from build123d import *


with BuildPart() as f1:
    # F0 (on Front) → F1 (revolve)
    with BuildSketch(Plane.XZ):
        Polygon((2.2225, 3.048), (2.2225, 0), (4.678082, 0), (4.826, 0.4064), (4.826, 1.143), (3.81, 1.143), (3.81, 1.778), (4.826, 4.569437), (4.826, 15.1384), (3.937, 16.3068), (3.937, 19.7104), (3.6068, 19.7104), (3.6068, 16.3068), (4.4958, 15.1384), (4.064, 4.064), (0.9398, 4.064), (0.9398, 3.048), align=None)
    revolve(axis=Axis((0, 0, 11.499301), (0, 0, 1)))


with BuildPart() as f2_1:
    # F2: copy of F1
    add(f1.part)


solid = f1.part
The model under review builds one solid part; all positions refer to its coordinate system, in mm. A direction names the side the tool comes from. Round coordinates to 2 decimals unless told otherwise and drop trailing zeros. Write each loop counter-clockwise with the first axis right and the second up, starting at its lowest first coordinate (ties: lowest second). Pieces come first, ordered by that corner, then holes. Notation, with made-up numbers: (69, 40.25) -> (97, 40.25) arc R17 ccw to (97, 62.25) -> close; hole circle Ø3 at (-4, 27). An arc over 180 degrees is marked (long way). Answer as a JSON object with one key per item and string values.
1. Clearance check with flat-ended pins moving along their axes: pin 1 (5 mm diameter, centred on y = -3.5, z = 5.5, fed in from +X); pin 2 (3 mm diameter, centred on x = 0, y = 0, fed in from +Z); pin 3 (1.5 mm diameter, centred on x = -3, z = 8, fed in from +Y); pin 4 (5 mm diameter, centred on x = 2.5, z = 4.5, fed in from -Y). State where each tip first meets the part, or that it passes through.
Results found:
{"pin 1": "stops at x = 4.72", "pin 2": "stops at z = 4.06", "pin 3": "stops at y = 4.27", "pin 4": "stops at y = -4.83"}
2. We need section C-C on z = 18. State the section outline as (x, y) points.
Results found:
{"outline": "circle Ø7.87 at (0, 0); hole circle Ø7.21 at (0, 0)"}
3. Machinability: for faces 5 (the face through (-0.48, -2.17, 1.5)), 6 (the face through (-0.83, -3.72, 1.46)), 7 (the face through (-3.83, -2.937, 9.928)), 8 (the face through (-0.853, -3.843, 18.032)), which of the approach directions +Z, -Z, +X, -X, +Y, -Y give a long, thin tool a straight path to every point of the face, cutting with its end or side? Answer none if there is none.
Results found:
{"face 5": "-Z", "face 6": "none", "face 7": "+Z, -Z", "face 8": "+Z"}
4. To check wall thickness, follow line 1 along Y through (x, z) = (0, 17.4); line 2 along Y through (x, z) = (1.5, 7.75); line 3 along Z through (x, y) = (0.75, 1.5). State the ranges of each line that lie inside material, in increasing order.
Results found:
{"line 1": "y = -3.94 to -3.61, 3.61 to 3.94", "line 2": "y = -4.59 to -3.93, 3.93 to 4.59", "line 3": "z = 3.05 to 4.06"}
5. We need section D-D on z = 7.75. State the section outline as (x, y) points.
Results found:
{"outline": "circle Ø9.65 at (0, 0); hole circle Ø8.42 at (0, 0)"}
6. The part is to be moulded in two halves that separate along X. For faces 1 (the face through (-0.2, -0.92, 3.55)), 2 (the face through (-3, -2, 18)), 3 (the face through (-3.83, -2.937, 0.78)), 4 (the face through (4, 1, 1.143)), say which applies: pulls with the +X half, pulls with the -X half, needs draft (parallel to the pull), parting line crosses it, or undercut.
Results found:
{"face 1": "undercut", "face 2": "undercut", "face 3": "parting line crosses it", "face 4": "needs draft"}
